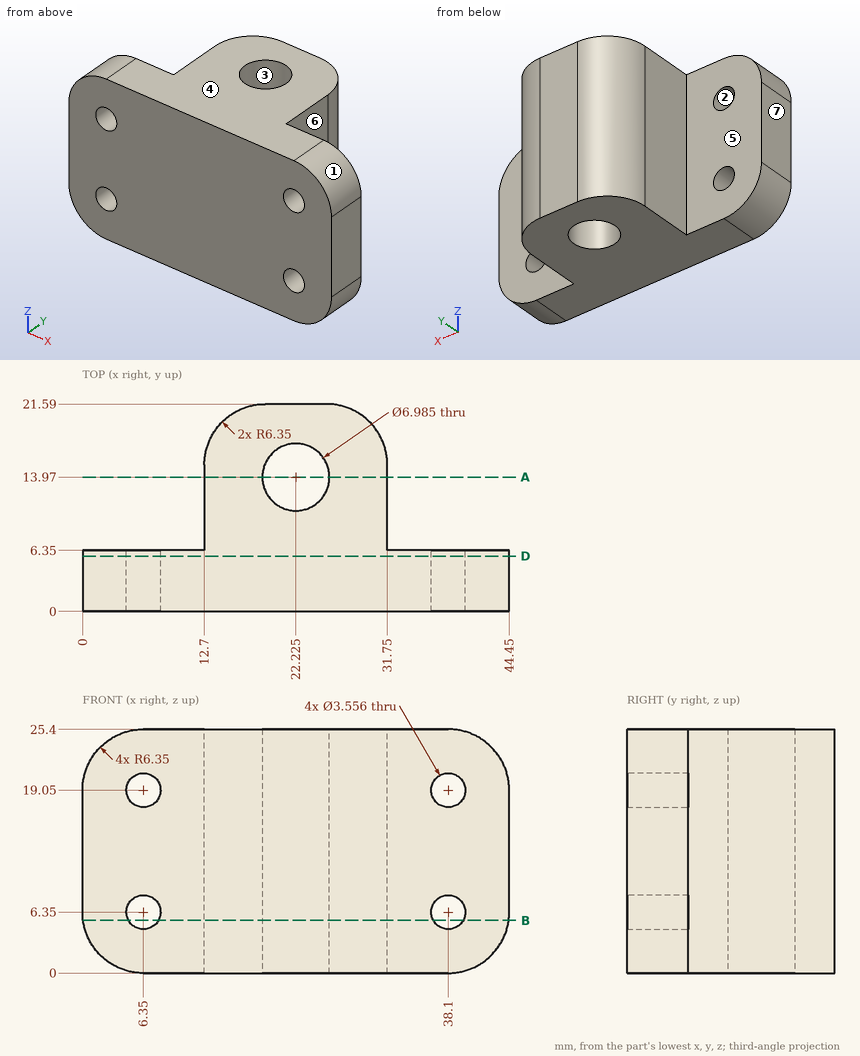
The drawing under review shows one solid part. Ordinate dimensions are in mm from its lowest x, y, z. A direction names the side the tool comes from. Give positions to 0.01 mm unless a question says otherwise; leave off trailing zeros. Write each loop counter-clockwise with the first axis right and the second up, starting at its lowest first coordinate (ties: lowest second). Pieces come first, ordered by that corner, then holes. Notation, with made-up numbers: (-39, 53.5) - (-35, 53.5) arc R14 cw to (-35, 69.5) - close; hole circle Ø3 at (89.5, -4.75). An arc over 180 degrees is marked (long way). Answer in a Markdown table with one row per item. Add a question column.
1. Tool access review of the marked faces 5, 6 and 7: name each direction out of +Z, -Z, +X, -X, +Y, -Y from which nothing blocks a thin tool from reaching the whole face with its end or side.
2. We need section D-D on y = 5.75. Write out the cut boundary in (x, z).
3. Wall thickness on line 1 along X through (y, z) = (4, 6.35); line 2 along X through (y, z) = (1, 7.25); line 3 along X through (y, z) = (8.25, 1.5): over which ranges is each line inside the solid? List them lowest first. Write a range as [from, to].
4. We need section A-A on y = 13.97. Write out the cut boundary in (x, z).
5. Draft analysis for pull direction X (two halves, no side actions). For the marked faces 1, 2, 3 and 4, state which applies: +X half, -X half, draft (parallel to the pull), parting line (faces both ways), or undercut.
6. Insertion check: P1, Ø10, axis at x = 4, z = 14, coming from the +Y side; P2, Ø2.5, axis at y = 10, z = 10.5, coming from the +X side; P3, Ø1.5, axis at y = 14, z = 6.5, coming from the -X side; P4, Ø1, axis at x = 38.5, y = 7.5, coming from the -Z side. Each pin has a flat end and moves straight along its axis. Give the tip position at first contact, or say it passes through.
7. We need section B-B on z = 5.5. State how many separate pieces and enclosed holes the cut face has, then the cut area to 3 significant figures.
Ans:
| question | item | result |
|---|---|---|
| 1 | face 5 | +Z, -Z, -X, +Y |
| 1 | face 6 | +Z, -Z, +X, +Y |
| 1 | face 7 | +Z, -Z, -X, +Y, -Y |
| 2 | outline | (0, 6.35) arc R6.35 ccw to (6.35, 0) - (38.1, 0) arc R6.35 ccw to (44.45, 6.35) - (44.45, 19.05) arc R6.35 ccw to (38.1, 25.4) - (6.35, 25.4) arc R6.35 ccw to (0, 19.05) - close; hole circle Ø3.56 at (6.35, 6.35); hole circle Ø3.56 at (6.35, 19.05); hole circle Ø3.56 at (38.1, 6.35); hole circle Ø3.56 at (38.1, 19.05) |
| 3 | line 1 | x = [0, 4.57], [8.13, 36.32], [39.88, 44.45] |
| 3 | line 2 | x = [0, 4.82], [7.88, 36.57], [39.63, 44.45] |
| 3 | line 3 | x = [12.7, 31.75] |
| 4 | outline | (12.7, 0) - (18.73, 0) - (18.73, 25.4) - (12.7, 25.4) - close; (25.72, 0) - (31.75, 0) - (31.75, 25.4) - (25.72, 25.4) - close |
| 5 | face 1 | +X half |
| 5 | face 2 | undercut |
| 5 | face 3 | undercut |
| 5 | face 4 | draft |
| 6 | P1 | stops at y = 6.35 |
| 6 | P2 | stops at x = 31.75 |
| 6 | P3 | stops at x = 12.7 |
| 6 | P4 | passes through |
| 7 | separate pieces | 3 |
| 7 | enclosed holes | 1 |
| 7 | area | 477 mm^2 |
